Autodesk Inventor part; units mm, degrees
ref_plane "YZ Plane" through (0, 0, 0) normal (1, 0, 0) x (0, 1, 0)
ref_plane "XZ Plane" through (0, 0, 0) normal (0, 1, 0) x (-1, 0, 0)
ref_plane "XY Plane" through (0, 0, 0) normal (0, 0, 1) x (1, 0, 0)
sketch "草圖1" plane through (0, 0, 0) normal (0, 0, 1) x (1, 0, 0)
  line L0 (0, 0) -> (0, 15)
  line L1 (0, 15) -> (45, 15)
  line L2 (45, 15) -> (45, 0)
  line L3 (45, 0) -> (37.5, 0)
  line L4 (37.5, 0) -> (37.5, 8)
  line L5 (37.5, 8) -> (7.5, 8)
  line L6 (7.5, 8) -> (7.5, 0)
  line L7 (7.5, 0) -> (0, 0)
  dimension "d0" = 15
  dimension "d1" = 8
  dimension "d2" = 30
  dimension "d3" = 45
  dimension "d4" = 7.5
extrude "擠出1" add sketch "草圖1" against normal blind 60
sketch "草圖2" plane through (0, 15, 0) normal (0, 1, 0) x (1, 0, 0)
  line L0 (15, 34) -> (15, 11)
  line L1 (30, 34) -> (30, 11)
  arc A0 (30, 34) -> (15, 34) centre (22.5, 34) ccw
  arc A1 (15, 11) -> (30, 11) centre (22.5, 11) ccw
  line L2 (0, 0) -> (45, 0)
  line L3 (0, 0) -> (0, 60)
  dimension "d7" = 11
  dimension "d8" = 15
  dimension "d9" = 7.5
  dimension "d10" = 23
  dimension "d11" = 7.5
  dimension "d12" = 22.5
extrude "擠出2" cut sketch "草圖2" against normal blind 7
sketch "草圖3" plane through (0, 0, -60) normal (0, 0, -1) x (-1, 0, 0)
  line L0 (-45, 15) -> (-45, 0)
  line L1 (-45, 15) -> (-45, 27)
  line L2 (-45, 27) -> (-34, 38)
  line L3 (-34, 38) -> (-11, 38)
  line L4 (-11, 38) -> (0, 27)
  line L5 (0, 27) -> (0, 15)
  line L6 (0, 15) -> (-45, 15)
  line L7 (0, 15) -> (-45, 15)
  circle A0 centre (-22.5, 26) radius 7.5
  line L8 (-7.5, 0) -> (0, 0)
  dimension "d15" = 11
  dimension "d16" = 11
  dimension "d17" = 11
  dimension "d18" = 11
  dimension "d19" = 38
  dimension "d20" = 11
  dimension "d21" = 15
  dimension "d22" = 22.5
extrude "擠出3" add sketch "草圖3" against normal blind 11
properties part number "410571040練習二"
Can you work these out from the model? Positions are in its coordinate system, mm. A direction names the side the tool comes from. Coordinates: 2 decimals unless noted, no trailing zeros. Loops run counter-clockwise (first coordinate to the right, second up) from the corner with the lowest first, then second, coordinate; pieces in that order, holes last. Notation, with made-up numbers: M 56,-19 L 65,-19 A15 cw 65,5 Z; hole C 82,-19.5 d2. An arc over 180 degrees is marked long. Put each result on its own line as item: value. Start each with the question number.
(1) Imagine slicing it at D-D on z = -51.5. List the corners of the cut face in (x, y) for me, and give its area (3 significant figures).
(2) We'd pull the mould along X, two halves only. Please class faces 5 (the face through (22.66, 11.55, -41.5)), 6 (the face through (18, 19, -49)), 7 (the face through (6, 33, -55)): +X half, -X half, draft (parallel to the pull), parting line (faces both ways), or undercut.
(3) Imagine slicing it at B-B on y = 3.5. List the corners of the cut face in (x, z) for me, and give its area (3 significant figures).
(4) Which directions (+Z, -Z, +X, -X, +Y, -Y) give clear straight access to the entire face, cutting with the end or side of a thin tool? Please do faces 1 (the face through (30, 12, -23)), 2 (the face through (12, 15, -24)), 3 (the face through (23, 38, -55)), 4 (the face through (7.5, 4, -30)).
(5) Imagine slicing it at C-C on x = 22.5. List the corners of the cut face in (y, z) for me.
(6) Will these pins go through, and if not, where does the flat tip stop? pin 1 Ø2.5 at (y, z) = (3.5, -18.5) entering from -X; pin 2 Ø6 at (x, z) = (23.5, -42.5) entering from +Y; pin 3 Ø9 at (x, z) = (18.5, -22) entering from -Y.
(7) Imagine slicing it at A-A on z = -5. List the corners of the cut face in (x, y) for me.
(8) I need wall thicknesses on probe 1 along X at (y, z) = (9, -26); probe 2 along X at (y, z) = (3.5, -35); probe 3 along Y at (x, z) = (22.5, -53.5). Which ranges of each line are inside material? Lowest first, please.
Worked answers:
1. outline: M 0,0 L 7.5,0 L 7.5,8 L 37.5,8 L 37.5,0 L 45,0 L 45,27 L 34,38 L 11,38 L 0,27 Z; hole C 22.5,26 d15
1. area: 1,170 mm2
2. face 5: undercut
2. face 6: draft
2. face 7: -X half
3. outline: M 0,-60 L 7.5,-60 L 7.5,0 L 0,0 Z; M 37.5,-60 L 45,-60 L 45,0 L 37.5,0 Z
3. area: 900 mm2
4. face 1: +Y, -Y
4. face 2: +Z, +X, -X, +Y
4. face 3: +Z, -Z, +X, -X, +Y
4. face 4: +Z, -Z, -Y
5. outline: M 8,-60 L 18.5,-60 L 18.5,-49 L 15,-49 L 15,-41.5 L 8,-41.5 Z; M 8,-3.5 L 15,-3.5 L 15,0 L 8,0 Z; M 33.5,-60 L 38,-60 L 38,-49 L 33.5,-49 Z
6. pin 1: stops at x = 0
6. pin 2: stops at y = 15
6. pin 3: stops at y = 8
7. outline: M 0,0 L 7.5,0 L 7.5,8 L 18,8 L 18,15 L 0,15 Z; M 27,8 L 37.5,8 L 37.5,0 L 45,0 L 45,15 L 27,15 Z
8. probe 1: x = 0 to 15, 30 to 45
8. probe 2: x = 0 to 7.5, 37.5 to 45
8. probe 3: y = 8 to 18.5, 33.5 to 38
